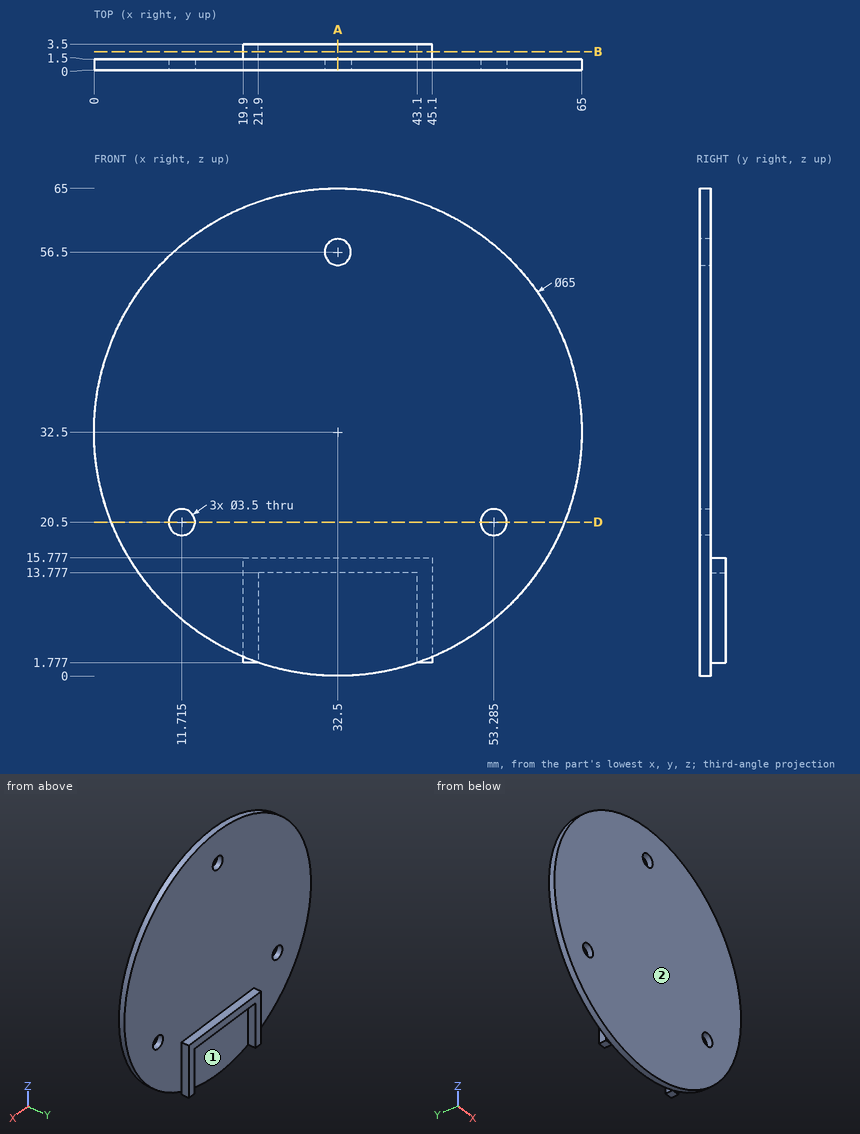
Job drawing, mm, ordinate dimensions from the low corner. One solid piece. Give positions to 0.01 mm unless a question says otherwise; leave off trailing zeros. Write each loop counter-clockwise with the first axis right and the second up, starting at its lowest first coordinate (ties: lowest second). Pieces come first, ordered by that corner, then holes. Notation, with made-up numbers: M 82,-38 L 90,-38 A13 cw 90,-21 Z; hole C -32,63.5 d11. An arc over 180 degrees is marked long. One line per item, written item: value. Start each with the question number.
Q1. Drop flat-ended pins along their axis: pin 1 Ø1 at (y, z) = (1.5, 36) entering from -X; pin 2 Ø2 at (x, y) = (21.5, 2) entering from -Z; pin 3 Ø2 at (x, z) = (32.5, 56.5) entering from +Y; pin 4 Ø1.6 at (y, z) = (2.5, 6.5) entering from -X. Give the stop position or say it passes through.
Q2. Saw through at D-D, the plane z = 20.5. Write the cut outline in (x, y) (1 decimal).
Q3. Saw through at B-B, the plane y = 2.5. Write the cut outline in (x, z).
Q4. Two-plate mould, pull along X, no slides. Class the marked faces 1 and 2: +X half, -X half, draft (parallel to the pull), parting line (faces both ways), or undercut.
Q5. Saw through at A-A, the plane x = 32.5. Write the cut outline in (y, z).
Q6. Probe probe 1 along X at (y, z) = (1.8, 13); probe 2 along Y at (x, z) = (60.5, 23.5); probe 3 along X at (y, z) = (0.2, 20). List the from-to ranges inside material, lowest first. Write a range as [from, to].
Output values:
1. pin 1: stops at x = 0.14
1. pin 2: stops at z = 1.62
1. pin 3: passes through
1. pin 4: stops at x = 19.9
2. outline: M 2.3,0 L 10,0 L 10,1.5 L 2.3,1.5 Z; M 13.5,0 L 51.5,0 L 51.5,1.5 L 13.5,1.5 Z; M 55,0 L 62.7,0 L 62.7,1.5 L 55,1.5 Z
3. outline: M 19.9,1.78 L 21.9,1.78 L 21.9,13.78 L 43.1,13.78 L 43.1,1.78 L 45.1,1.78 L 45.1,15.78 L 19.9,15.78 Z
4. face 1: undercut
4. face 2: draft
5. outline: M 0,0 L 1.5,0 L 1.5,13.78 L 3.5,13.78 L 3.5,15.78 L 1.5,15.78 L 1.5,54.75 L 0,54.75 Z; M 0,58.25 L 1.5,58.25 L 1.5,65 L 0,65 Z
6. probe 1: x = [19.9, 21.9], [43.1, 45.1]
6. probe 2: y = [0, 1.5]
6. probe 3: x = [2.5, 10.04], [13.39, 51.61], [54.96, 62.5]
